```python
from build123d import *

# Parameters (mm, degrees)
BOSS_EXTRUDE1_DEPTH = 332
SKETCH2_R           = 7.5
CUT_EXTRUDE1_DEPTH  = 330
SKETCH3_R           = 11
CUT_EXTRUDE2_DEPTH  = 5


with BuildPart() as part:
    # Sketch1 → Boss-Extrude1 (new body)
    with BuildSketch(Plane.XY):
        with BuildLine():
            Line((22.479289941, 29.51183432), (-35.520710059, 29.51183432))
            ThreePointArc((-35.520710059, 29.51183432), (-39.763350746, 27.754475007), (-41.520710059, 23.51183432))
            Line((-41.520710059, 23.51183432), (-41.520710059, -34.48816568))
            ThreePointArc((-41.520710059, -34.48816568), (-39.763350746, -38.730806368), (-35.520710059, -40.48816568))
            Line((-35.520710059, -40.48816568), (22.479289941, -40.48816568))
            ThreePointArc((22.479289941, -40.48816568), (26.721930628, -38.730806368), (28.479289941, -34.48816568))
            Line((28.479289941, -34.48816568), (28.479289941, 23.51183432))
            ThreePointArc((28.479289941, 23.51183432), (26.721930628, 27.754475007), (22.479289941, 29.51183432))
        make_face()
        with BuildLine():
            Line((22.479289941, 26.51183432), (-35.520710059, 26.51183432))
            ThreePointArc((-35.520710059, 26.51183432), (-37.642030403, 25.633154663), (-38.520710059, 23.51183432))
            Line((-38.520710059, 23.51183432), (-38.520710059, -34.48816568))
            ThreePointArc((-38.520710059, -34.48816568), (-37.642030403, -36.609486024), (-35.520710059, -37.48816568))
            Line((-35.520710059, -37.48816568), (22.479289941, -37.48816568))
            ThreePointArc((22.479289941, -37.48816568), (24.600610284, -36.609486024), (25.479289941, -34.48816568))
            Line((25.479289941, -34.48816568), (25.479289941, 23.51183432))
            ThreePointArc((25.479289941, 23.51183432), (24.600610284, 25.633154663), (22.479289941, 26.51183432))
        make_face(mode=Mode.SUBTRACT)
    extrude(amount=BOSS_EXTRUDE1_DEPTH)

    # Sketch2 → Cut-Extrude1 (cut)
    with BuildSketch(Plane(origin=(28.479289941, 0, 0), x_dir=(0, 0, -1), z_dir=(1, 0, 0))):
        with Locations(Location((-220.9, -5.48816568, 0), (0, 0, 90))):
            Circle(SKETCH2_R)
        with Locations(Location((-110.9, -5.48816568, 0), (0, 0, 90))):
            Circle(SKETCH2_R)
        Polygon((0, -40.48816568), (-13.6, 29.51183432), (0, 29.51183432), align=None)
        Polygon((-332, -40.48816568), (-332, 29.51183432), (-318.4, 29.51183432), align=None)
    extrude(amount=-CUT_EXTRUDE1_DEPTH, mode=Mode.SUBTRACT)

    # Sketch3 → Cut-Extrude2 (cut)
    with BuildSketch(Plane(origin=(28.479289941, 0, 0), x_dir=(0, 0, -1), z_dir=(1, 0, 0))):
        with Locations(Location((-220.9, -5.48816568, 0), (0, 0, 90))):
            Circle(SKETCH3_R)
        with Locations(Location((-110.9, -5.48816568, 0), (0, 0, 90))):
            Circle(SKETCH3_R)
    extrude(amount=-CUT_EXTRUDE2_DEPTH, mode=Mode.SUBTRACT)


solid = part.part
```
Geometry check sheet. Reference: the model listing, model coordinates, mm. A direction names the side the tool comes from. Coordinates: 2 decimals unless noted, no trailing zeros. Order: outer loops, then holes, each group sorted by start corner. A loop starts at its lowest first (then second) coordinate and runs counter-clockwise, first axis right, second up.
Item 1: Section check D-D (y = 12.5). Enter the section's corners in (x, z).
Item 2: Mould release check, pull along Z, two halves, no side actions. Record for faces 4 (the flat face through (27.346, -5.325, 325.168)), 5 (the cylindrical face through (26.768, 27.708, 163.85)), 6 (the cylindrical face through (27, -0.412, 211.141)): released by +Z, released by -Z, zero draft, split by the parting line, or undercut.
Item 3: Depth check by flat-ended pin: pin 1 (17 mm diameter, centred on y = -5.49, z = 220.9, fed in from +X). Enter the tip coordinate at first touch or a pass-through.
Item 4: Section check C-C (z = 220.9). Enter the section's corners in (x, y).
Item 5: Section check A-A (z = 187). Enter the section's corners in (x, y), plus the area to 3 significant figures.
Item 6: Scan lines: line 1 along Y through (x, z) = (-26.5, 163); line 2 along X through (y, z) = (15.5, 27); line 3 along X through (y, z) = (-36.5, 156.5). Record each from-to range of solid material in increasing order.
Item 7: Tool access check on faces 1 (the cylindrical face through (27, -7.87, 100.16)), 2 (the flat face through (28.479, -6, 164)), 3 (the flat face through (-38.521, -5, 164)). Record the directions out of +Z, -Z, +X, -X, +Y, -Y that give a thin tool (end or side, any length) a straight path to the whole face; none if there is none.
Item 8: Section check B-B (y = -9). Enter the section's corners in (x, z).
Check sheet entries:
1. outline: (-41.52, 10.29) - (-38.52, 10.29) - (-38.52, 321.71) - (-41.52, 321.71) - close; (25.48, 10.29) - (28.48, 10.29) - (28.48, 321.71) - (25.48, 321.71) - close
2. face 4: released by +Z
2. face 5: zero draft
2. face 6: undercut
3. pin 1: stops at x = -38.52
4. outline: (-41.52, -34.49) arc R6 ccw to (-35.52, -40.49) - (22.48, -40.49) arc R6 ccw to (28.48, -34.49) - (28.48, -16.49) - (25.48, -16.49) - (25.48, -34.49) arc R3 cw to (22.48, -37.49) - (-35.52, -37.49) arc R3 cw to (-38.52, -34.49) - (-38.52, -12.99) - (-41.52, -12.99) - close; (-41.52, 2.01) - (-38.52, 2.01) - (-38.52, 23.51) arc R3 cw to (-35.52, 26.51) - (22.48, 26.51) arc R3 cw to (25.48, 23.51) - (25.48, 5.51) - (28.48, 5.51) - (28.48, 23.51) arc R6 ccw to (22.48, 29.51) - (-35.52, 29.51) arc R6 ccw to (-41.52, 23.51) - close
5. outline: (-41.52, -34.49) arc R6 ccw to (-35.52, -40.49) - (22.48, -40.49) arc R6 ccw to (28.48, -34.49) - (28.48, 23.51) arc R6 ccw to (22.48, 29.51) - (-35.52, 29.51) arc R6 ccw to (-41.52, 23.51) - close; hole (-38.52, -34.49) arc R3 ccw to (-35.52, -37.49) - (22.48, -37.49) arc R3 ccw to (25.48, -34.49) - (25.48, 23.51) arc R3 ccw to (22.48, 26.51) - (-35.52, 26.51) arc R3 ccw to (-38.52, 23.51) - close
5. area: 781 mm2
6. line 1: y = -40.49 to -37.49, 26.51 to 29.51
6. line 2: x = -41.52 to -38.52, 25.48 to 28.48
6. line 3: x = -41.17 to -37.75, 24.7 to 28.13
7. face 1: +X
7. face 2: +Z, -Z, +X, +Y, -Y
7. face 3: +Z, -Z
8. outline: (-41.52, 6.12) - (-38.52, 6.12) - (-38.52, 104.27) - (-41.52, 104.27) - close; (-41.52, 117.53) - (-38.52, 117.53) - (-38.52, 214.27) - (-41.52, 214.27) - close; (-41.52, 227.53) - (-38.52, 227.53) - (-38.52, 325.88) - (-41.52, 325.88) - close; (25.48, 6.12) - (28.48, 6.12) - (28.48, 100.48) - (25.48, 100.48) - close; (25.48, 121.32) - (28.48, 121.32) - (28.48, 210.48) - (25.48, 210.48) - close; (25.48, 231.32) - (28.48, 231.32) - (28.48, 325.88) - (25.48, 325.88) - close
